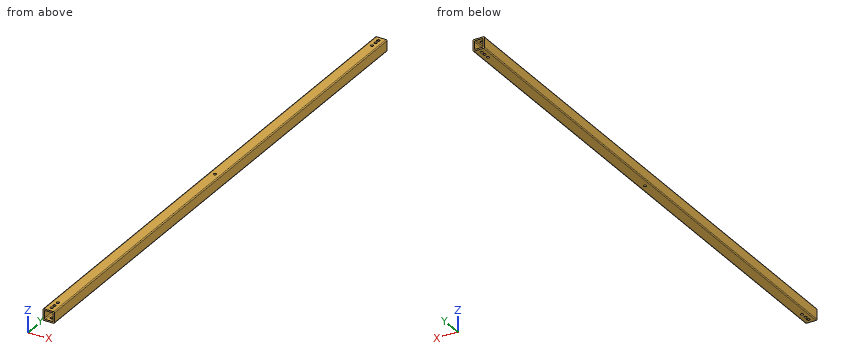
from build123d import *

# Parameters (mm, degrees)
SKETCH1_W           = 25.4
SKETCH1_H           = 25.4
SKETCH1_W_2         = 19.05
SKETCH1_H_2         = 19.05
BOSS_EXTRUDE1_DEPTH = 609.6
FILLET1_R           = 2.1082
SKETCH6_R           = 3.175
CUT_EXTRUDE5_DEPTH  = 611.261099858
SKETCH7_R           = 3.175
CUT_EXTRUDE6_DEPTH  = 611.261099858


with BuildPart() as part:
    # Sketch1 → Boss-Extrude1 (new, symmetric)
    with BuildSketch(Plane(origin=(0, 0, 0), x_dir=(1, 0, 0), z_dir=(0, 1, 0))):
        Rectangle(SKETCH1_W, SKETCH1_H)
        Rectangle(SKETCH1_W_2, SKETCH1_H_2, mode=Mode.SUBTRACT)
    extrude(amount=BOSS_EXTRUDE1_DEPTH, both=True)

    # Fillet1
    fillet1_edges = [part.edges().sort_by_distance(p)[0] for p in [
        (9.525, 0, 9.525),
        (9.525, 0, -9.525),
        (-9.525, 0, -9.525),
        (-9.525, 0, 9.525),
        (-12.7, 0, -12.7),
        (12.7, 0, -12.7),
        (12.7, 0, 12.7),
        (-12.7, 0, 12.7),
    ]]
    fillet(fillet1_edges, radius=FILLET1_R)

    # Sketch6 → Cut-Extrude5 (cut, through all)
    with BuildSketch(Plane(origin=(0, 0, -12.7), x_dir=(-1, 0, 0), z_dir=(0, 0, -1))):
        with Locations((0, -598.805)):
            Circle(SKETCH6_R)
        with Locations((0, -588.645)):
            Circle(SKETCH6_R)
        with Locations((0, -575.945)):
            Circle(SKETCH6_R)
        with Locations((0, 598.805)):
            Circle(SKETCH6_R)
        with Locations((0, 588.645)):
            Circle(SKETCH6_R)
        with Locations((0, 575.945)):
            Circle(SKETCH6_R)
    extrude(amount=-CUT_EXTRUDE5_DEPTH, mode=Mode.SUBTRACT)

    # Sketch7 → Cut-Extrude6 (cut, through all)
    with BuildSketch(Plane(origin=(0, 0, -12.7), x_dir=(-1, 0, 0), z_dir=(0, 0, -1))):
        Circle(SKETCH7_R)
    extrude(amount=-CUT_EXTRUDE6_DEPTH, mode=Mode.SUBTRACT)


solid = part.part
Could you check a few things on this model? Use its own coordinates, in mm. Coordinates: 2 decimals unless noted, no trailing zeros. Write each loop counter-clockwise with the first axis right and the second up, starting at its lowest first coordinate (ties: lowest second). Pieces come first, ordered by that corner, then holes. Notation, with made-up numbers: (-11, 4.25) - (46, 4.25) arc R17 ccw to (46, 8.25) - close; hole circle Ø8 at (-21, -5). An arc over 180 degrees is marked (long way). Write item = value, one per line.
1) Suppose I cut it at A-A on z = 0.75. Please give me the cut outline in (x, y) (3 decimals), plus the area to 3 significant figures.
Result set:
outline = (-12.7, -609.6) - (-9.525, -609.6) - (-9.525, 609.6) - (-12.7, 609.6) - close; (9.525, -609.6) - (12.7, -609.6) - (12.7, 609.6) - (9.525, 609.6) - close
area = 7,740 mm2
2) Suppose I cut it at B-B on y = 214. Please give me the cut outline in (x, z) (3 decimals).
Result set:
outline = (-12.7, -10.592) arc R2.108 ccw to (-10.592, -12.7) - (10.592, -12.7) arc R2.108 ccw to (12.7, -10.592) - (12.7, 10.592) arc R2.108 ccw to (10.592, 12.7) - (-10.592, 12.7) arc R2.108 ccw to (-12.7, 10.592) - close; hole (-9.525, -7.417) arc R2.108 ccw to (-7.417, -9.525) - (7.417, -9.525) arc R2.108 ccw to (9.525, -7.417) - (9.525, 7.417) arc R2.108 ccw to (7.417, 9.525) - (-7.417, 9.525) arc R2.108 ccw to (-9.525, 7.417) - close
3) Please list where these lines run through material, in increasing order: line 1 (Z direction, x = -4, y = -35) (3 decimals); line 2 (X direction, y = -296, z = -10.75). Write a range as [from, to].
Result set:
line_1 = [-12.7, -9.525], [9.525, 12.7]
line_2 = [-12.69, 12.69]
